Design review of the part built by this model. Coordinates are the model's own, in mm. A direction names the side the tool comes from. Coordinates: 2 decimals unless noted, no trailing zeros. Loops run counter-clockwise (first coordinate to the right, second up) from the corner with the lowest first, then second, coordinate; pieces in that order, holes last. Notation, with made-up numbers: (87.5, -25.75) -> (138.5, -25.75) arc R16 cw to (138.5, 1.25) -> close; hole circle Ø1 at (10, -13.5). An arc over 180 degrees is marked (long way). Use CSV: the item, a comma, the result in double quotes.
```python
from build123d import *

# Parameters (mm, degrees)
SKETCH1_R           = 13.97
BOSS_EXTRUDE2_DEPTH = 50.8
SKETCH2_R           = 29.718
BOSS_EXTRUDE3_DEPTH = 3.175
SKETCH3_R           = 25.4
BOSS_EXTRUDE4_DEPTH = 8.382
SKETCH4_R           = 13.97
BOSS_EXTRUDE5_DEPTH = 101.6
SKETCH5_R           = 10.842824112
CUT_EXTRUDE1_DEPTH  = 101.6


with BuildPart() as part:
    # Sketch1 → Boss-Extrude2 (new body)
    with BuildSketch(Plane.XY):
        Circle(SKETCH1_R)
    extrude(amount=BOSS_EXTRUDE2_DEPTH)

    # Sketch2 → Boss-Extrude3 (add)
    with BuildSketch(Plane.XY.offset(50.8)):
        Circle(SKETCH2_R)
    extrude(amount=BOSS_EXTRUDE3_DEPTH)

    # Sketch3 → Boss-Extrude4 (add)
    with BuildSketch(Plane.XY.offset(53.975)):
        Circle(SKETCH3_R)
    extrude(amount=BOSS_EXTRUDE4_DEPTH)

    # Sketch4 → Boss-Extrude5 (add)
    with BuildSketch(Plane.XY.offset(62.357)):
        Circle(SKETCH4_R)
    extrude(amount=BOSS_EXTRUDE5_DEPTH)

    # Sketch5 → Cut-Extrude1 (cut)
    with BuildSketch(Plane.XY.offset(163.957)):
        Circle(SKETCH5_R)
    extrude(amount=-CUT_EXTRUDE1_DEPTH, mode=Mode.SUBTRACT)


solid = part.part
```
Item 1: Add section D-D (z = 42). Give the boundary of the cut face in (x, y), then the cut area to 3 significant figures.
Checked values:
outline,"circle Ø27.94 at (0, 0)"
area,"613 mm^2"
Item 2: Clearance check with flat-ended pins moving along their axes: pin 1 (2 mm diameter, centred on y = 1.5, z = 132.5, fed in from -X); pin 2 (4 mm diameter, centred on y = -14.5, z = 111.5, fed in from +X); pin 3 (6 mm diameter, centred on y = 12.5, z = 52.5, fed in from +X); pin 4 (10 mm diameter, centred on x = -20.5, z = 79, fed in from -Y). State where each tip first meets the part, or that it passes through.
Checked values:
pin 1,"x = -13.96"
pin 2,"x = 6.24"
pin 3,"x = 28.16"
pin 4,"through"
Item 3: Add section A-A (x = 0). Give the boundary of the cut face in (y, z) (3 decimals).
Checked values:
outline,"(-29.718, 50.8) -> (-13.97, 50.8) -> (-13.97, 0) -> (13.97, 0) -> (13.97, 50.8) -> (29.718, 50.8) -> (29.718, 53.975) -> (25.4, 53.975) -> (25.4, 62.357) -> (13.97, 62.357) -> (13.97, 163.957) -> (10.843, 163.957) -> (10.843, 62.357) -> (-10.843, 62.357) -> (-10.843, 163.957) -> (-13.97, 163.957) -> (-13.97, 62.357) -> (-25.4, 62.357) -> (-25.4, 53.975) -> (-29.718, 53.975) -> close"
Item 4: Add section B-B (z = 117.5). Give the boundary of the cut face in (x, y), then the cut area to 3 significant figures.
Checked values:
outline,"circle Ø27.94 at (0, 0); hole circle Ø21.69 at (0, 0)"
area,"244 mm^2"
Item 5: Draft analysis for pull direction X (two halves, no side actions). For faces 3 (the face through (6, -13, 50.8)), 4 (the face through (0, 0, 62.357)), 5 (the face through (-1.82, 13.85, 25.04)), state which applies: pulls with the +X half, pulls with the -X half, needs draft (parallel to the pull), parting line crosses it, or undercut.
Checked values:
face 3,"needs draft"
face 4,"undercut"
face 5,"parting line crosses it"
Item 6: Machinability: for faces 1 (the face through (0, 0, 0)), 2 (the face through (22, 13, 53.975)), which of the approach directions +Z, -Z, +X, -X, +Y, -Y give a long, thin tool a straight path to every point of the face, cutting with its end or side? Answer none if there is none.
Checked values:
face 1,"-Z, +X, -X, +Y, -Y"
face 2,"+Z"
Item 7: To check wall thickness, follow line 1 along Y through (x, z) = (0, 110); line 2 along Z through (x, y) = (11, -23) (3 decimals); line 3 along Y through (x, z) = (9, 154). State the ranges of each line that lie inside material, in increasing order.
Checked values:
line 1,"-13.97 to -10.84, 10.84 to 13.97"
line 2,"50.8 to 53.975"
line 3,"-10.68 to -6.05, 6.05 to 10.68"
